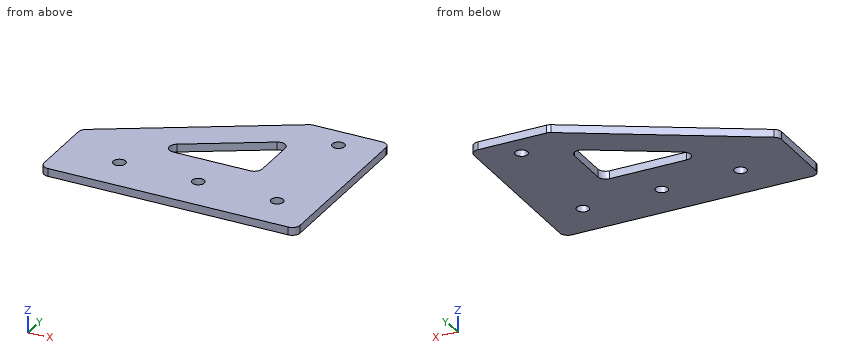
from build123d import *

# Parameters (mm, degrees)
EXTRUDE_1_DEPTH     = 2
SKETCH_2_R          = 1.55
CUT_EXTRUDE_1_DEPTH = 3
FILLET_1_R          = 2


with BuildPart() as part:
    # 草图1 → 凸台-拉伸1 (new body)
    with BuildSketch(Plane.XY):
        Polygon((-55, -180), (10, -180), (10, -134.019237886), (-10, -134.019237886), (-55, -160), align=None)
    extrude(amount=EXTRUDE_1_DEPTH)

    # 草图2 → 切除-拉伸1 (cut, through all)
    with BuildSketch(Plane(origin=(0, 0, 0), x_dir=(-1, 0, 0), z_dir=(0, 0, -1))):
        with Locations((40, -170)):
            Circle(SKETCH_2_R)
        with Locations((20, -170)):
            Circle(SKETCH_2_R)
        with Locations((0, -170)):
            Circle(SKETCH_2_R)
        with Locations((0, -140)):
            Circle(SKETCH_2_R)
        with BuildLine():
            Line((12, -160), (31.535898385, -160))
            ThreePointArc((31.535898385, -160), (33.467750037, -158.51763809), (32.535898385, -156.267949192))
            Line((32.535898385, -156.267949192), (13, -144.988893001))
            ThreePointArc((13, -144.988893001), (11, -144.988893001), (10, -146.720943809))
            Line((10, -146.720943809), (10, -158))
            ThreePointArc((10, -158), (10.585786438, -159.414213562), (12, -160))
        make_face()
    extrude(amount=-CUT_EXTRUDE_1_DEPTH, mode=Mode.SUBTRACT)

    # 圆角1
    fillet_1_edges = [part.edges().sort_by_distance(p)[0] for p in [
        (-55, -160, 1),
        (-10, -134.019237886, 1),
        (10, -134.019237886, 1),
        (10, -180, 1),
        (-55, -180, 1),
    ]]
    fillet(fillet_1_edges, radius=FILLET_1_R)


solid = part.part
Work out the finished part from the listing and answer in its coordinate system (mm). Give positions to 0.01 mm unless a question says otherwise; leave off trailing zeros. Loops run counter-clockwise (first coordinate to the right, second up) from the corner with the lowest first, then second, coordinate; pieces in that order, holes last. Notation, with made-up numbers: (6.5, -27) -> (39.5, -27) arc R19 ccw to (39.5, 9) -> close; hole circle Ø9 at (84.25, 88). An arc over 180 degrees is marked (long way). Use a Markdown table: item, result. Add a question column.
1) Consider line 1 along X through (y, z) = (-170, 0.75); line 2 along Y through (x, z) = (-20, 0.5); line 3 along X through (y, z) = (-154.5, 0.65). Determine where each line is inside the solid, lowest interval first.
2) The part is cut by section D-D, the plane y = -140. Determine the outline of the cut face in (x, z).
3) The part is cut by section A-A, the plane x = 0. Determine the outline of the cut face in (y, z).
4) The part is cut by section C-C, the plane z = 1.5. Determine the outline of the cut face in (x, y).
5) The part is cut by section B-B, the plane y = -170. Determine the outline of the cut face in (x, z).
6) Each of these flat-tipped pins is pushed along its axis until it touches: P1, Ø3.5, axis at x = 0, y = -170, coming from the -Z side; P2, Ø0.6, axis at y = -153, z = 1, coming from the -X side; P3, Ø1, axis at x = -21.5, z = 0.5, coming from the +Y side. Where does it stop, or does it pass through?
Reported:
| question | item | result |
|---|---|---|
| 1 | line 1 | x = -55 to -41.55, -38.45 to -21.55, -18.45 to -1.55, 1.55 to 10 |
| 1 | line 2 | y = -180 to -171.55, -168.45 to -160, -149.03 to -139.79 |
| 1 | line 3 | x = -45.47 to -29.47, -10 to 10 |
| 2 | outline | (-20.36, 0) -> (-1.55, 0) -> (-1.55, 2) -> (-20.36, 2) -> close; (1.55, 0) -> (10, 0) -> (10, 2) -> (1.55, 2) -> close |
| 3 | outline | (-180, 0) -> (-171.55, 0) -> (-171.55, 2) -> (-180, 2) -> close; (-168.45, 0) -> (-141.55, 0) -> (-141.55, 2) -> (-168.45, 2) -> close; (-138.45, 0) -> (-134.02, 0) -> (-134.02, 2) -> (-138.45, 2) -> close |
| 4 | outline | (-55, -178) arc R2 ccw to (-53, -180) -> (8, -180) arc R2 ccw to (10, -178) -> (10, -136.02) arc R2 ccw to (8, -134.02) -> (-9.46, -134.02) arc R2 ccw to (-10.46, -134.29) -> (-54, -159.42) arc R2 ccw to (-55, -161.15) -> close; hole circle Ø3.1 at (-40, -170); hole (-32.54, -156.27) arc R2 ccw to (-31.54, -160) -> (-12, -160) arc R2 ccw to (-10, -158) -> (-10, -146.72) arc R2 ccw to (-13, -144.99) -> close; hole circle Ø3.1 at (-20, -170); hole circle Ø3.1 at (0, -170); hole circle Ø3.1 at (0, -140) |
| 5 | outline | (-55, 0) -> (-41.55, 0) -> (-41.55, 2) -> (-55, 2) -> close; (-38.45, 0) -> (-21.55, 0) -> (-21.55, 2) -> (-38.45, 2) -> close; (-18.45, 0) -> (-1.55, 0) -> (-1.55, 2) -> (-18.45, 2) -> close; (1.55, 0) -> (10, 0) -> (10, 2) -> (1.55, 2) -> close |
| 6 | P1 | stops at z = 0 |
| 6 | P2 | stops at x = -43.4 |
| 6 | P3 | stops at y = -140.37 |
